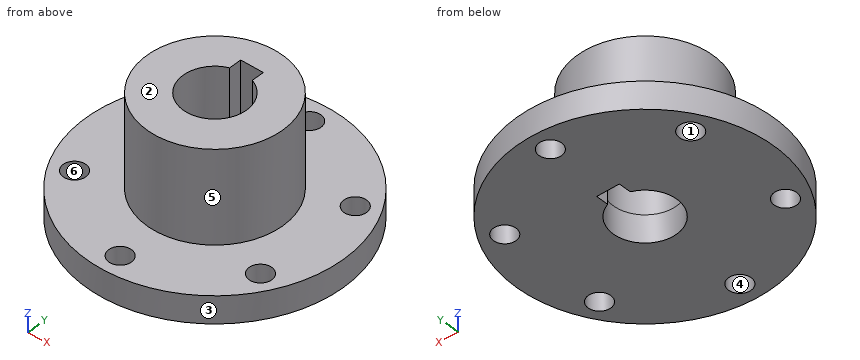
Autodesk Inventor part; units mm, degrees
ref_plane "YZ Plane" through (0, 0, 0) normal (1, 0, 0) x (0, 1, 0)
ref_plane "XZ Plane" through (0, 0, 0) normal (0, 1, 0) x (-1, 0, 0)
ref_plane "XY Plane" through (0, 0, 0) normal (0, 0, 1) x (1, 0, 0)
sketch "Base" plane through (0, 0, 0) normal (0, 0, 1) x (1, 0, 0)
  circle A0 centre (0, 0) radius 28.4
  circle A1 centre (0, 0) radius 23.75 construction
  circle A2 centre (0, 0) radius 7
  line L0 (-2.5, 0) -> (2.5, 0)
  line L1 (2.5, 0) -> (2.5, 9.3)
  line L2 (2.5, 9.3) -> (-2.5, 9.3)
  line L3 (-2.5, 9.3) -> (-2.5, 0)
  line L4 (0, -39.76) -> (0, 39.76) construction
  circle A3 centre (0, 23.75) radius 2.5
  circle A4 centre (-20.5681, 11.875) radius 2.5
  circle A5 centre (-20.5681, -11.875) radius 2.5
  circle A6 centre (0, -23.75) radius 2.5
  circle A7 centre (20.5681, -11.875) radius 2.5
  circle A8 centre (20.5681, 11.875) radius 2.5
  point P0 (0, 9.3)
  point P1 (2.5, 6.5383)
  point P2 (-2.5, 6.5383)
  dimension "d1" = 47.5
  dimension "d0" = 56.8
  dimension "d2" = 14
  dimension "d3" = 9.3
  dimension "d4" = 5
  dimension "d5" = 5
  dimension "d8" = 360
extrude "BaseFeature" add sketch "Base" along normal blind 6
sketch "Lip" plane through (0, 0, 6) normal (0, 0, 1) x (1, 0, 0)
  arc A0 (-2.5, 6.5383) -> (2.5, 6.5383) centre (0, 0) ccw
  circle A1 centre (0, 0) radius 15
  line L0 (-2.5, 6.5383) -> (-2.5, 9.3)
  line L1 (2.5, 9.3) -> (2.5, 6.5383)
  line L2 (-2.5, 9.3) -> (2.5, 9.3)
  dimension "d12" = 30
extrude "LipFeature" add sketch "Lip" along normal blind 20.4
properties part number "NexusRobot14mmKeywayHub"
Geometry: final body of the model. Coordinates: model frame, mm. Face numbers are marked on the shaded views. A direction names the side the tool comes from. Coordinates: 2 decimals unless noted, no trailing zeros. Order: outer loops, then holes, each group sorted by start corner. A loop starts at its lowest first (then second) coordinate and runs counter-clockwise, first axis right, second up.
1) Section A-A (y = 4.5). Return loops of the section in (x, z), then the cut area to 3 significant figures.
Result sheet:
outline: (-28.04, 0) - (-5.36, 0) - (-5.36, 26.4) - (-14.31, 26.4) - (-14.31, 6) - (-28.04, 6) - close; (5.36, 0) - (28.04, 0) - (28.04, 6) - (14.31, 6) - (14.31, 26.4) - (5.36, 26.4) - close
area: 637 mm2
2) Section B-B (z = 4.25). Return loops of the section in (x, y) (3 decimals), then the cut area to 3 significant figures.
Result sheet:
outline: circle Ø56.8 at (0, 0); hole circle Ø5 at (-20.568, -11.875); hole circle Ø5 at (-20.568, 11.875); hole circle Ø5 at (0, -23.75); hole (-2.5, 6.538) arc R7 ccw (long way) to (2.5, 6.538) - (2.5, 9.3) - (-2.5, 9.3) - close; hole circle Ø5 at (0, 23.75); hole circle Ø5 at (20.568, -11.875); hole circle Ø5 at (20.568, 11.875)
area: 2,250 mm2
3) Section D-D (x = 20). Return loops of the section in (y, z), then the cut area to 3 significant figures.
Result sheet:
outline: (-20.16, 0) - (-14.31, 0) - (-14.31, 6) - (-20.16, 6) - close; (-9.44, 0) - (9.44, 0) - (9.44, 6) - (-9.44, 6) - close; (14.31, 0) - (20.16, 0) - (20.16, 6) - (14.31, 6) - close
area: 184 mm2
4) Set-up query: the marked faces 5 and 6. Return all of +Z, -Z, +X, -X, +Y, -Y with unobstructed straight access to the full face (end or side cutting, diameter ignored); none if empty.
Result sheet:
face 5: +Z
face 6: +Z, -Z
5) First-contact query: P1, Ø4, axis at y = 9, z = 23.5, coming from the +X side; P2, Ø8, axis at x = 0, y = 23.75, coming from the -Z side; P3, Ø5, axis at x = 17.5, y = -20.5, coming from the +Z side; P4, Ø10, axis at x = -18, z = 8, coming from the +Y side. Flat tips, straight axial feed; report the tip coordinate or a pass-through.
Result sheet:
P1: stops at x = 13.27
P2: stops at z = 0
P3: stops at z = 6
P4: stops at y = 25.03
6) Draft query along Y for the marked faces 1, 2, 3 and 4. Return one class per face: released by +Y, released by -Y, zero draft, split by the parting line, or undercut.
Result sheet:
face 1: undercut
face 2: zero draft
face 3: split by the parting line
face 4: undercut
7) Section C-C (x = 0). Return loops of the section in (y, z).
Result sheet:
outline: (-28.4, 0) - (-26.25, 0) - (-26.25, 6) - (-28.4, 6) - close; (-21.25, 0) - (-7, 0) - (-7, 26.4) - (-15, 26.4) - (-15, 6) - (-21.25, 6) - close; (9.3, 0) - (21.25, 0) - (21.25, 6) - (15, 6) - (15, 26.4) - (9.3, 26.4) - close; (26.25, 0) - (28.4, 0) - (28.4, 6) - (26.25, 6) - close
8) Ray query, probe 1 along Y at (x, z) = (0, 1.7); probe 2 along Y at (x, z) = (0, 19.5); probe 3 along Y at (x, z) = (-18.5, 1.5). Return the intervals inside material, ascending.
Result sheet:
probe 1: y = -28.4 to -26.25, -21.25 to -7, 9.3 to 21.25, 26.25 to 28.4
probe 2: y = -15 to -7, 9.3 to 15
probe 3: y = -21.55 to -13.28, -10.47 to 10.47, 13.28 to 21.55
